from build123d import *

# Parameters (mm, degrees)
SKETCH1_W           = 20
SKETCH1_H           = 44
SKETCH1_R           = 2.1
BOSS_EXTRUDE1_DEPTH = 5
SKETCH2_R           = 2.1
CUT_EXTRUDE1_DEPTH  = 3


with BuildPart() as part:
    # Sketch1 → Boss-Extrude1 (new body)
    with BuildSketch(Plane(origin=(0, 0, 0), x_dir=(1, 0, 0), z_dir=(0, 1, 0))):
        with Locations((0, -0.5)):
            Rectangle(SKETCH1_W, SKETCH1_H)
        with Locations((0, -13.5)):
            Circle(SKETCH1_R, mode=Mode.SUBTRACT)
        with Locations((0, 13.5)):
            Circle(SKETCH1_R, mode=Mode.SUBTRACT)
        with Locations((0, -44.5)):
            Rectangle(SKETCH1_W, SKETCH1_H)
        with Locations((0, -58.5)):
            Circle(SKETCH1_R, mode=Mode.SUBTRACT)
        with Locations((0, -31.5)):
            Circle(SKETCH1_R, mode=Mode.SUBTRACT)
    extrude(amount=BOSS_EXTRUDE1_DEPTH)

    # Sketch2 → Cut-Extrude1 (cut)
    with BuildSketch(Plane(origin=(0, 5, 0), x_dir=(1, 0, 0), z_dir=(0, 1, 0))):
        Polygon((0, 17.6), (3.6, 15.6), (-3.6, 15.6), align=None)
        with BuildLine():
            ThreePointArc((2.1, 13.5), (1.48492424, 12.01507576), (0, 11.4))
            Line((0, 11.4), (3.6, 11.4))
            Line((3.6, 11.4), (3.6, 15.6))
            Line((3.6, 15.6), (0, 15.6))
            ThreePointArc((0, 15.6), (1.48492424, 14.98492424), (2.1, 13.5))
        make_face()
        with BuildLine():
            Line((-3.6, 15.6), (-3.6, 11.4))
            Line((-3.6, 11.4), (0, 11.4))
            ThreePointArc((0, 11.4), (-2.1, 13.5), (0, 15.6))
            Line((0, 15.6), (-3.6, 15.6))
        make_face()
        Polygon((0, 9.4), (-3.6, 11.4), (3.6, 11.4), align=None)
        Polygon((0, -9.4), (3.6, -11.4), (-3.6, -11.4), align=None)
        with BuildLine():
            ThreePointArc((2.1, -13.5), (1.484924244, -14.984924237), (1e-08, -15.6))
            Line((1e-08, -15.6), (3.6, -15.6))
            Line((3.6, -15.6), (3.6, -11.4))
            Line((3.6, -11.4), (0, -11.4))
            ThreePointArc((0, -11.4), (1.48492424, -12.01507576), (2.1, -13.5))
        make_face()
        with BuildLine():
            Line((-3.6, -11.4), (-3.6, -15.6))
            Line((-3.6, -15.6), (1e-08, -15.6))
            ThreePointArc((1e-08, -15.6), (-2.1, -13.500000005), (0, -11.4))
            Line((0, -11.4), (-3.6, -11.4))
        make_face()
        Polygon((0, -17.6), (-3.6, -15.6), (3.6, -15.6), align=None)
        Polygon((0, -35.6), (-3.6, -33.6), (-3.6, -29.4), (0, -27.4), (3.6, -29.4), (3.6, -33.6), align=None)
        with Locations((0, -31.5)):
            Circle(SKETCH2_R, mode=Mode.SUBTRACT)
        Polygon((0, -62.6), (-3.6, -60.6), (-3.6, -56.4), (0, -54.4), (3.6, -56.4), (3.6, -60.6), align=None)
        with Locations((0, -58.5)):
            Circle(SKETCH2_R, mode=Mode.SUBTRACT)
    extrude(amount=-CUT_EXTRUDE1_DEPTH, mode=Mode.SUBTRACT)


solid = part.part
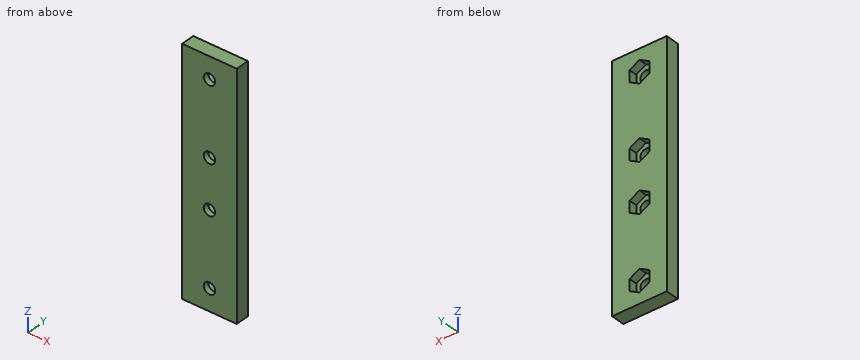
Geometry check sheet. Reference: the model listing, model coordinates, mm. Coordinates: 2 decimals unless noted, no trailing zeros. Write each loop counter-clockwise with the first axis right and the second up, starting at its lowest first coordinate (ties: lowest second). Pieces come first, ordered by that corner, then holes. Notation, with made-up numbers: (64.25, 6) -> (75.25, 6) arc R21 ccw to (75.25, 20) -> close; hole circle Ø9 at (-27.75, 32.5). An arc over 180 degrees is marked (long way). One line per question, with ' | ' between items.
1. Thickness scan on probe 1 along Z at (x, y) = (0, 0.95); probe 2 along X at (y, z) = (1.4, 13.5); probe 3 along X at (y, z) = (4.3, 34.5). Record the ranges inside material, lowest first. Write a range as from..to.
Answers:
probe 1: z = -21.5..-15.6, -11.4..11.4, 15.6..29.4, 33.6..56.4, 60.6..66.5 | probe 2: x = -10..-2.1, 2.1..10 | probe 3: x = -10..-1.98, 1.98..10
2. Cross-section at A-A on y = 3.7. Record the cut outline in (x, z).
Answers:
outline: (-10, -21.5) -> (10, -21.5) -> (10, 66.5) -> (-10, 66.5) -> close; hole (-3.6, -15.6) -> (0, -17.6) -> (3.6, -15.6) -> (3.6, -11.4) -> (0, -9.4) -> (-3.6, -11.4) -> close; hole (-3.6, 11.4) -> (0, 9.4) -> (3.6, 11.4) -> (3.6, 15.6) -> (0, 17.6) -> (-3.6, 15.6) -> close; hole (-3.6, 29.4) -> (0, 27.4) -> (3.6, 29.4) -> (3.6, 33.6) -> (0, 35.6) -> (-3.6, 33.6) -> close; hole (-3.6, 56.4) -> (0, 54.4) -> (3.6, 56.4) -> (3.6, 60.6) -> (0, 62.6) -> (-3.6, 60.6) -> close
3. Depth check by flat-ended pin: pin 1 Ø2.5 at (x, z) = (0, 31.5) entering from -Y (1 decimal); pin 2 Ø3.5 at (x, z) = (0, 30.5) entering from +Y. Enter the tip coordinate at first touch or a pass-through.
Answers:
pin 1: passes through | pin 2: stops at y = 2
4. Cross-section at B-B on z = 13.5. Record the cut outline in (x, y).
Answers:
outline: (-10, 0) -> (-2.1, 0) -> (-2.1, 2) -> (-3.6, 2) -> (-3.6, 5) -> (-10, 5) -> close; (2.1, 0) -> (10, 0) -> (10, 5) -> (3.6, 5) -> (3.6, 2) -> (2.1, 2) -> close
5. Cross-section at C-C on x = 0.75. State how many separate pieces and enclosed holes the cut face has, and give its area (3 significant figures).
Answers:
separate pieces: 5 | enclosed holes: 0 | area: 320 mm²
